```python
from build123d import *

# Parameters (mm, degrees)
EXTRUDE_THIN1_DEPTH = 421.049210887
FILLET1_R           = 10
SKETCH_2_R          = 19.05
EXTRUDE_1_DEPTH     = 23.24974156
SKETCH_3_R          = 19.05
EXTRUDE_2_DEPTH     = 23


with BuildPart() as part:
    # Sketch1 → Extrude-Thin1 (new body, symmetric)
    with BuildSketch(Plane.XY):
        Polygon((-250.514148937, 25.753634758), (-250.514148937, 0), (440.503291061, 0), (440.503291061, 25.915671281), (446.551474959, 25.915671281), (446.551474959, -6.048183898), (-256.562332835, -6.048183898), (-256.562332835, 25.753634758), align=None)
    extrude(amount=EXTRUDE_THIN1_DEPTH, both=True)

    # Fillet1
    fillet1_edges = [part.edges().sort_by_distance(p)[0] for p in [
        (-253.538240886, 25.753634758, 421.049210887),
        (443.52738301, 25.915671281, 421.049210887),
        (-253.538240886, 25.753634758, -421.049210887),
        (443.52738301, 25.915671281, -421.049210887),
    ]]
    fillet(fillet1_edges, radius=FILLET1_R)

    # 草图2 → 凸台-拉伸1 (add)
    with BuildSketch(Plane(origin=(0, -6.048183898, 0), x_dir=(-1, 0, 0), z_dir=(0, -1, 0))):
        with Locations((-360.164689426, 358.012657815)):
            Circle(SKETCH_2_R)
    extrude(amount=EXTRUDE_1_DEPTH)

    # 草图3 → 凸台-拉伸2 (add)
    with BuildSketch(Plane(origin=(0, -6.048183898, 0), x_dir=(-1, 0, 0), z_dir=(0, -1, 0))):
        with Locations((174.06050089, -351.274172881)):
            Circle(SKETCH_3_R)
    extrude(amount=EXTRUDE_2_DEPTH)


solid = part.part
```
Can you work these out from the model? Positions are in its coordinate system, mm. A direction names the side the tool comes from. Round coordinates to 2 decimals unless told otherwise and drop trailing zeros. Loops run counter-clockwise (first coordinate to the right, second up) from the corner with the lowest first, then second, coordinate; pieces in that order, holes last. Notation, with made-up numbers: (36, 3) -> (72, 3) arc R9 ccw to (72, 7) -> close; hole circle Ø5 at (-14, 14.5). An arc over 180 degrees is marked (long way). One line per item, written item: value. Start each with the question number.
1. If we section it at B-B, the plane y = -18: Write out the boundary of the cut face in (x, z), then the cut area to 3 significant figures.
2. If we mould it in two halves opening along X, with no side actions, what happens to faces 1 (the flat face through (-250.514, 13, 6)), 2 (the flat face through (446.551, 10, 6)), 3 (the cylindrical face through (-192.23, -17.39, 345.55))? For each: pulls with the +X half, pulls with the -X half, needs draft (parallel to the pull), parting line crosses it, or undercut.
3. If we section it at D-D, the plane x = -172.5: Write out the boundary of the cut face in (y, z), then the cut area to 3 significant figures.
4. For pin 1 (5 mm diameter, centred on x = 351, z = -265, fed in from -Y); pin 2 (8 mm diameter, centred on x = 75.5, z = -264, fed in from +Y); pin 3 (11.5 mm diameter, centred on x = -178, z = 356, fed in from -Y), each with a flat end and sliding along its axis, tell me the tip position at first contact or that it passes through.
5. For faces 4 (the cylindrical face through (349.924, -17.51, -374.076)), 5 (the flat face through (-256.562, 10, 6)), 6 (the flat face through (440.503, 13, 6)), which set-ups out of +Z, -Z, +X, -X, +Y, -Y let a thin tool reach every point of the face, with its end or its side?
6. If we section it at A-A, the plane z = -102.5: Write out the boundary of the cut face in (x, y).
7. If we section it at C-C, the plane x = 94.5: Write out the boundary of the cut face in (y, z).
8. If I drill on probe 1 along X at (y, z) = (9.5, 387); probe 2 along Y at (x, z) = (316, -295); probe 3 along X at (y, z) = (-7.5, 340), over which ranges is the centre line in solid material (lowest first)?
Calculated:
1. outline: circle Ø38.1 at (-174.06, 351.27); circle Ø38.1 at (360.16, -358.01)
1. area: 2,280 mm²
2. face 1: undercut
2. face 2: pulls with the +X half
2. face 3: parting line crosses it
3. outline: (-29.05, 332.29) -> (-6.05, 332.29) -> (-6.05, -421.05) -> (0, -421.05) -> (0, 421.05) -> (-6.05, 421.05) -> (-6.05, 370.26) -> (-29.05, 370.26) -> close
3. area: 5,970 mm²
4. pin 1: stops at y = -6.05
4. pin 2: stops at y = 0
4. pin 3: stops at y = -29.05
5. face 4: -Y
5. face 5: +Z, -Z, -X, +Y, -Y
5. face 6: +Z, -Z, +Y
6. outline: (-256.56, -6.05) -> (446.55, -6.05) -> (446.55, 25.92) -> (440.5, 25.92) -> (440.5, 0) -> (-250.51, 0) -> (-250.51, 25.75) -> (-256.56, 25.75) -> close
7. outline: (-6.05, -421.05) -> (0, -421.05) -> (0, 421.05) -> (-6.05, 421.05) -> close
8. probe 1: x = -256.56 to -250.51, 440.5 to 446.55
8. probe 2: y = -6.05 to 0
8. probe 3: x = -189.42 to -158.7
